```python
from build123d import *

# Parameters (mm, degrees)
SKETCH_W     = 64
SKETCH_H     = 114
PAD_DEPTH    = 13
SKETCH002_W  = 58
SKETCH002_H  = 108
POCKET_DEPTH = 11
SKETCH007_W  = 2.5
SKETCH007_H  = 2.5
PAD001_DEPTH = 3
FILLET_R     = 1.5


with BuildPart() as part:
    # Sketch → Pad (new body)
    with BuildSketch(Plane.XY):
        with Locations((4.5, 30)):
            Rectangle(SKETCH_W, SKETCH_H)
    extrude(amount=PAD_DEPTH)

    # Sketch002 → Pocket (cut)
    with BuildSketch(Plane.XY.offset(13)):
        with Locations((4.5, 30)):
            Rectangle(SKETCH002_W, SKETCH002_H)
    extrude(amount=-POCKET_DEPTH, mode=Mode.SUBTRACT)

    # Sketch007 → Pad001 (new body)
    with BuildSketch(Plane.XY.offset(2)):
        with Locations((-18, 77.5)):
            Rectangle(SKETCH007_W, SKETCH007_H)
        with Locations((27, 77.5)):
            Rectangle(SKETCH007_W, SKETCH007_H)
        with Locations((-18, -17.5)):
            Rectangle(SKETCH007_W, SKETCH007_H)
        with Locations((27, -17.5)):
            Rectangle(SKETCH007_W, SKETCH007_H)
    extrude(amount=PAD001_DEPTH)

    # Fillet
    fillet_edges = [part.edges().sort_by_distance(p)[0] for p in [
        (4.5, 87, 0),
        (-27.5, 30, 0),
        (36.5, 30, 0),
        (4.5, -27, 0),
    ]]
    fillet(fillet_edges, radius=FILLET_R)


solid = part.part
```
For this review, take the finished solid that the model builds, in its own axes (mm). A direction names the side the tool comes from. Give positions to 0.01 mm unless a question says otherwise; leave off trailing zeros. Write each loop counter-clockwise with the first axis right and the second up, starting at its lowest first coordinate (ties: lowest second). Pieces come first, ordered by that corner, then holes.
Item 1: Wall thickness on probe 1 along X at (y, z) = (45, 11.75); probe 2 along Y at (x, z) = (-16, 10); probe 3 along Z at (x, y) = (-8, 55.5): over which ranges is each line inside the solid? List them lowest first.
Item 2: Take a section at C-C (y = -1). Give the boundary of the cut face in (x, z), and give its area (3 significant figures).
Item 3: Insertion check: P1, Ø0.8, axis at x = -17.5, y = -17, coming from the +Z side; P2, Ø1, axis at x = -13.5, y = 13, coming from the +Z side. Each pin has a flat end and moves straight along its axis. Give the tip position at first contact, or say it passes through.
Item 4: The part is to be moulded in two halves that separate along Y. For faces 3 (the face through (-27.5, 29, 7)), 4 (the face through (-19.25, -18, 3)), 5 (the face through (4, 87, 7)), say which applies: +Y half, -Y half, draft (parallel to the pull), parting line (faces both ways), or undercut.
Item 5: Machinability: for faces 1 (the face through (4, -27, 7)), 2 (the face through (25.75, 77, 3)), which of the approach directions +Z, -Z, +X, -X, +Y, -Y give a long, thin tool a straight path to every point of the face, cutting with its end or side? Answer none if there is none.
Item 6: Take a section at B-B (x = 15). Give the boundary of the cut face in (y, z), and give its area (3 significant figures).
Item 7: Take a section at A-A (z = 3.75). Give the boundary of the cut face in (x, y).
Established:
1. probe 1: x = -27.5 to -24.5, 33.5 to 36.5
1. probe 2: y = -27 to -24, 84 to 87
1. probe 3: z = 0 to 2
2. outline: (-27.5, 1.5) arc R1.5 ccw to (-26, 0) - (35, 0) arc R1.5 ccw to (36.5, 1.5) - (36.5, 13) - (33.5, 13) - (33.5, 2) - (-24.5, 2) - (-24.5, 13) - (-27.5, 13) - close
2. area: 193 mm2
3. P1: stops at z = 5
3. P2: stops at z = 2
4. face 3: draft
4. face 4: undercut
4. face 5: +Y half
5. face 1: +Z, -Z, +X, -X, -Y
5. face 2: +Z
6. outline: (-27, 1.5) arc R1.5 ccw to (-25.5, 0) - (85.5, 0) arc R1.5 ccw to (87, 1.5) - (87, 13) - (84, 13) - (84, 2) - (-24, 2) - (-24, 13) - (-27, 13) - close
6. area: 293 mm2
7. outline: (-27.5, -27) - (36.5, -27) - (36.5, 87) - (-27.5, 87) - close; (-19.25, -18.75) - (-16.75, -18.75) - (-16.75, -16.25) - (-19.25, -16.25) - close; (-19.25, 76.25) - (-16.75, 76.25) - (-16.75, 78.75) - (-19.25, 78.75) - close; (25.75, -18.75) - (28.25, -18.75) - (28.25, -16.25) - (25.75, -16.25) - close; (25.75, 76.25) - (28.25, 76.25) - (28.25, 78.75) - (25.75, 78.75) - close; hole (-24.5, -24) - (33.5, -24) - (33.5, 84) - (-24.5, 84) - close
